The model under review builds one solid part; all positions refer to its coordinate system, in mm. Give positions to 0.01 mm unless a question says otherwise; leave off trailing zeros. Order: outer loops, then holes, each group sorted by start corner. A loop starts at its lowest first (then second) coordinate and runs counter-clockwise, first axis right, second up. Notation, with made-up numbers: (-34.5, -35.75) - (16.5, -35.75) arc R14 cw to (16.5, -25.75) - close; hole circle Ø2 at (74.5, 83). An arc over 180 degrees is marked (long way). Use CSV: the item, a comma, the result in double quotes. Start each with the question number.
1. Take a section at A-A, the plane y = 10. State the section outline as (x, z) points.
2. Take a section at B-B, the plane z = 6.35. State the section outline as (x, y) points.
3. Draft analysis for pull direction Z (two halves, no side actions). For faces 1 (the flat face through (1, 82, 12.7)), 2 (the cylindrical face through (1.48, 11.33, 5.66)), 3 (the flat face through (0, 80, 6)), state which applies: released by +Z, released by -Z, zero draft, split by the parting line, or undercut.
4. To check wall thickness, follow line 1 (Y direction, x = 1.7, z = 6.35); line 2 (Z direction, x = 2.1, y = 22.5) (3 decimals); line 3 (Z direction, x = 1.6, y = 10). State the ranges of each line that lie inside material, in increasing order. Write a range as [from, to].
5. For pin 1 (1 mm diameter, centred on x = 1, y = 30, fed in from -Z), flat-tipped, find the tip position at first contact; note if it passes through.
Autodesk Inventor part; units mm, degrees
ref_plane "YZ Plane" through (0, 0, 0) normal (1, 0, 0) x (0, 1, 0)
ref_plane "XZ Plane" through (0, 0, 0) normal (0, 1, 0) x (-1, 0, 0)
ref_plane "XY Plane" through (0, 0, 0) normal (0, 0, 1) x (1, 0, 0)
sketch "Skizze1" plane through (0, 0, 0) normal (1, 0, 0) x (0, 1, 0)
  line L0 (0, 0) -> (161.813, 0)
  line L1 (161.813, 0) -> (161.813, 12.7)
  line L2 (161.813, 12.7) -> (0, 12.7)
  line L3 (0, 12.7) -> (0, 0)
  dimension "d0" = 161.813
  dimension "d1" = 12.7
extrude "Extrusion1" add sketch "Skizze1" along normal blind 3
sketch "Skizze4" plane through (3, 0, 0) normal (1, 0, 0) x (0, 0, -1)
  line L0 (-12.7, 0) -> (0, 0)
  line L1 (-6.35, 0) -> (-6.35, 22.5)
  line L2 (-6.35, 0) -> (16.15, 0) construction
  line L3 (-6.35, 22.5) -> (-9.525, 22.5)
  line L4 (-6.35, 22.5) -> (-3.175, 22.5)
  line L5 (0, 161.813) -> (-12.7, 161.813)
  line L6 (-6.35, 161.813) -> (-6.35, 139.313)
  line L7 (-6.35, 139.313) -> (-9.525, 139.313)
  line L8 (-6.35, 139.313) -> (-3.175, 139.313)
  dimension "d16" = 22.5
  dimension "d17" = 90
  dimension "d18" = 3.175
  dimension "d19" = 3.175
  dimension "d20" = 22.5
  dimension "d21" = 3.175
  dimension "d22" = 3.175
hole "Bohrung2" at (3, 22.5, 9.525) at (3, 22.5, 3.175) at (3, 139.313, 9.525) at (3, 139.313, 3.175) direction (-1, 0, 0) diameter 1 end through all
sketch "Skizze5" plane through (3, 0, 0) normal (1, 0, 0) x (0, 0, -1)
  line L0 (-12.7, 0) -> (0, 0)
  line L1 (-6.35, 0) -> (-6.35, 10)
  line L2 (0, 161.813) -> (-12.7, 161.813)
  line L3 (-6.35, 161.813) -> (-6.35, 151.813)
  dimension "d30" = 10
  dimension "d31" = 10
hole "Bohrung3" at (3, 10, 6.35) at (3, 151.813, 6.35) direction (-1, 0, 0) diameter 3 end through all
properties part number "Platte_Kettenglied_unten"
Determined:
1,outline,"(0, 0) - (3, 0) - (3, 4.85) - (0, 4.85) - close; (0, 7.85) - (3, 7.85) - (3, 12.7) - (0, 12.7) - close"
2,outline,"(0, 0) - (3, 0) - (3, 8.5) - (0, 8.5) - close; (0, 11.5) - (3, 11.5) - (3, 150.31) - (0, 150.31) - close; (0, 153.31) - (3, 153.31) - (3, 161.81) - (0, 161.81) - close"
3,face 1,"released by +Z"
3,face 2,"undercut"
3,face 3,"zero draft"
4,line 1,"y = [0, 8.5], [11.5, 150.31], [153.31, 161.81]"
4,line 2,"z = [0, 2.675], [3.675, 9.025], [10.025, 12.7]"
4,line 3,"z = [0, 4.85], [7.85, 12.7]"
5,pin 1,"stops at z = 0"
